Check sheet for the modelled part. Datum: model origin and axes. Units: mm. A direction names the side the tool comes from. Round coordinates to 2 decimals unless told otherwise and drop trailing zeros. Loops run counter-clockwise (first coordinate to the right, second up) from the corner with the lowest first, then second, coordinate; pieces in that order, holes last. Notation, with made-up numbers: (-27.5, 61) -> (-10.5, 61) arc R23 cw to (-10.5, 90) -> close; hole circle Ø11 at (22.5, -1). An arc over 180 degrees is marked (long way). Return JSON: item names as keys, results as strings.
Autodesk Inventor part; units mm, degrees
ref_plane "YZ Plane" through (0, 0, 0) normal (1, 0, 0) x (0, 1, 0)
ref_plane "XZ Plane" through (0, 0, 0) normal (0, 1, 0) x (-1, 0, 0)
ref_plane "XY Plane" through (0, 0, 0) normal (0, 0, 1) x (1, 0, 0)
sketch "Sketch1" plane through (0, 0, 0) normal (0, 1, 0) x (-1, 0, 0)
  circle A0 centre (0, 0) radius 5
  dimension "d0" = 10
extrude "Extrusion1" add sketch "Sketch1" along normal blind 65
sketch "Sketch2" plane through (0, 65, 0) normal (0, 1, 0) x (1, 0, 0)
  circle A0 centre (0, 0) radius 5
  dimension "d38" = 10
chamfer "Chamfer1" distance 1 angle 45 1 edges at (5, 65, 0)
extrude "Extrusion2" add sketch "Sketch2" along normal blind 30
chamfer "Chamfer2" distance 1 angle 45 1 edges at (-5, 65, 0)
sketch "Sketch3" plane through (0, 0, 0) normal (0, -1, 0) x (1, 0, 0)
  line L0 (0, 0) -> (0, 0) construction
  line L1 (4.5, -7.7942) -> (-4.5, -7.7942)
  line L2 (-4.5, -7.7942) -> (-9, 0)
  line L3 (-9, 0) -> (-4.5, 7.7942)
  line L4 (-4.5, 7.7942) -> (4.5, 7.7942)
  line L5 (4.5, 7.7942) -> (9, 0)
  line L6 (9, 0) -> (4.5, -7.7942)
  circle A0 centre (0, 0) radius 5
  line L7 (-4.5, -7.7942) -> (4.5, 7.7942) construction
  line L8 (-4.5, 7.7942) -> (4.5, -7.7942) construction
  dimension "d21" = 9
  dimension "d22" = 9
  dimension "d23" = 120
  dimension "d24" = 9
  dimension "d25" = 9
  dimension "d26" = 120
  dimension "d34" = 9
  dimension "d36" = 0
  dimension "d37" = 0
extrude "Extrusion3" add sketch "Sketch3" along normal blind 5 contours L1 L2 L3 L4 L5 L6 | A0
chamfer "Chamfer3" distance 1 angle 45 6 edges at (0, -5, -7.7942) (-6.75, -5, -3.8971) (-6.75, -5, 3.8971) (0, -5, 7.7942) (6.75, -5, 3.8971) (6.75, -5, -3.8971)
fillet "Fillet1" radius 1 12 edges at (-4.2113, -4.5, -7.2942) (4.2113, -4.5, -7.2942) (8.4226, -4.5, 0) (4.2113, -4.5, 7.2942) (-4.2113, -4.5, 7.2942) (-8.4226, -4.5, 0) (-5.884, -5, -3.3971) (-5.884, -5, 3.3971) (0, -5, 6.7942) (5.884, -5, 3.3971) (5.884, -5, -3.3971) (0, -5, -6.7942)
fillet "Fillet2" radius 1 12 edges at (4.5, -1.9543, -7.7942) (9, -1.9543, 0) (4.5, -1.9543, 7.7942) (-4.5, -1.9543, 7.7942) (-9, -1.9543, 0) (-4.5, -1.9543, -7.7942) (-6.75, 0, 3.8971) (-6.75, 0, -3.8971) (0, 0, 7.7942) (6.75, 0, 3.8971) (6.75, 0, -3.8971) (0, 0, -7.7942)
thread "Thread3"
equation "\"d21\" = d24"
equation "\"d22\" = d24"
equation "\"d25\" = d24"
properties part number "CIM Mount Bolt" material "Aluminum 6061-AHC"
Q1. Go/stop test with flat-tipped pins: pin 1 (10 mm diameter, centred on x = -3, y = 84, fed in from -Z); pin 2 (6 mm diameter, centred on x = -4, y = 16.5, fed in from +Z); pin 3 (4 mm diameter, centred on x = 2, y = 32.5, fed in from +Z). Record where each tip stops, or that it passes through.
Results list:
{"pin 1": "z = -5", "pin 2": "z = 4.9", "pin 3": "z = 5"}
Q2. Material ranges on line 1 (Y direction, x = -2.25, z = 7); line 2 (Z direction, x = -0.25, y = 62); line 3 (Y direction, x = 0.75, z = -5.75), recorded low to high.
Results list:
{"line 1": "-4.78 to -0.02", "line 2": "-4.99 to 4.99", "line 3": "-5 to 0"}
Q3. Tool access check on faces 1 (the cylindrical face through (-1.08, 80.3, -4.88)), 2 (the flat face through (-6.468, -4.359, -3.668)). Record the directions out of +Z, -Z, +X, -X, +Y, -Y that give a thin tool (end or side, any length) a straight path to the whole face; none if there is none.
Results list:
{"face 1": "+Y", "face 2": "-Z, -X, -Y"}
Q4. Section check B-B (y = 15). Record the boundary of the cut face in (x, z), then the cut area to 3 significant figures.
Results list:
{"outline": "circle Ø10 at (0, 0)", "area": "78.5 mm^2"}
